Could you check a few things on this model? Use its own coordinates, in mm. Face numbers are marked on the shaded views. A direction names the side the tool comes from. Coordinates: 2 decimals unless noted, no trailing zeros. Order: outer loops, then holes, each group sorted by start corner. A loop starts at its lowest first (then second) coordinate and runs counter-clockwise, first axis right, second up. Notation, with made-up numbers: (-9.75, -20.5) -> (17.25, -20.5) arc R26 cw to (17.25, -4.5) -> close; hole circle Ø3 at (-33, 57). An arc over 180 degrees is marked (long way). Use a Markdown table: item, result. Add a question column.
1) If we section it at A-A (x = -27): Write out the boundary of the cut face in (y, z).
2) Will this pin go through, and if not, where does the flat tip stop? pin 1 Ø10 at (x, y) = (-1, -31) entering from +Z.
3) If we section it at B-B (z = 27): Write out the boundary of the cut face in (x, y).
4) If we section it at C-C (y = -5): Write out the boundary of the cut face in (x, z), plus the area to 3 significant figures.
5) Thinking about a two-plate mould opening in X: for the marked faces 4, 5, 6 and 7, which applies, +X half, -X half, draft (parallel to the pull), parting line (faces both ways), or undercut?
6) Which directions (+Z, -Z, +X, -X, +Y, -Y) give clear straight access to the entire face, cutting with the end or side of a thin tool? Please do the marked faces 1, 2 and 3.
7) If I drill on L1, parallel to Y at x = 35, z = 44.5; L2, parallel to X at y = -16, z = 49.5; L3, parallel to Z at x = -12, y = -6, over which ranges is the centre line in solid material (lowest first)? Write a range as [from, to].
```python
from build123d import *

# Parameters (mm, degrees)
F0_W     = 99.06
F0_H     = 71.12
F1_DEPTH = 71.12
F2_W     = 41.91
F2_H     = 27.94
F3_DEPTH = 66.04
F4_W     = 20.32
F4_H     = 3.81
F5_DEPTH = 10.16


with BuildPart() as f1:
    # F0 (on Top) → F1 (new body)
    with BuildSketch(Plane.XY):
        with Locations((0, -1.696959)):
            Rectangle(F0_W, F0_H)
    extrude(amount=F1_DEPTH)

    # F2 (on face) → F3 (cut)
    with BuildSketch(Plane.XY.offset(71.12)):
        with Locations((-20.955, 13.97)):
            Rectangle(F2_W, F2_H)
        with Locations((20.955, 13.97)):
            Rectangle(F2_W, F2_H)
        with Locations((20.955, -13.97)):
            Rectangle(F2_W, F2_H)
        with Locations((-20.955, -13.97)):
            Rectangle(F2_W, F2_H)
    extrude(amount=-F3_DEPTH, mode=Mode.SUBTRACT)

    # F4 (on face) → F5 (cut)
    with BuildSketch(Plane.XZ.offset(37.256959)):
        with Locations((0, 69.215)):
            Rectangle(F4_W, F4_H)
    extrude(amount=-F5_DEPTH, mode=Mode.SUBTRACT)


solid = f1.part
```
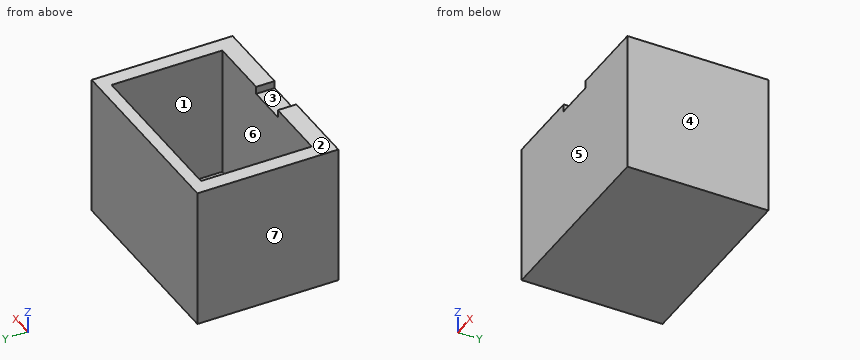
Answer sheet:
| question | item | result |
|---|---|---|
| 1 | outline | (-37.26, 0) -> (33.86, 0) -> (33.86, 71.12) -> (27.94, 71.12) -> (27.94, 5.08) -> (-27.94, 5.08) -> (-27.94, 71.12) -> (-37.26, 71.12) -> close |
| 2 | pin 1 | z = 67.31 |
| 3 | outline | (-49.53, -37.26) -> (49.53, -37.26) -> (49.53, 33.86) -> (-49.53, 33.86) -> close; hole (-41.91, -27.94) -> (41.91, -27.94) -> (41.91, 27.94) -> (-41.91, 27.94) -> close |
| 4 | outline | (-49.53, 0) -> (49.53, 0) -> (49.53, 71.12) -> (41.91, 71.12) -> (41.91, 5.08) -> (-41.91, 5.08) -> (-41.91, 71.12) -> (-49.53, 71.12) -> close |
| 4 | area | 1,510 mm2 |
| 5 | face 4 | +X half |
| 5 | face 5 | draft |
| 5 | face 6 | undercut |
| 5 | face 7 | -X half |
| 6 | face 1 | +Z |
| 6 | face 2 | +Z, +X, -X, +Y, -Y |
| 6 | face 3 | +Z, -Y |
| 7 | L1 | [-37.26, -27.94], [27.94, 33.86] |
| 7 | L2 | [-49.53, -41.91], [41.91, 49.53] |
| 7 | L3 | [0, 5.08] |
